```python
from build123d import *

# Parameters (mm, degrees)
BOX548_W               = 15
BOX548_H               = 13
BOX548_DEPTH           = 4.5
BOX548_ROLL_ANGLE      = 45
CYLINDER061_R          = 1.2
CYLINDER061_DEPTH      = 20
CYLINDER064_R          = 2
CYLINDER064_DEPTH      = 5
CYLINDER063_R          = 2
CYLINDER063_DEPTH      = 5
CYLINDER060_R          = 1.2
CYLINDER060_DEPTH      = 20
CYLINDER059_R          = 1.25
CYLINDER059_DEPTH      = 4.5
CYLINDER052_R          = 3.5
CYLINDER052_DEPTH      = 4.5
BOX043_W               = 7
BOX043_H               = 7.5
BOX043_DEPTH           = 5
BOX044_W               = 7
BOX044_H               = 7.5
BOX044_DEPTH           = 5
BOX041_W               = 8
BOX041_H               = 25
BOX041_DEPTH           = 4.5
CYLINDER053_R          = 5
CYLINDER053_DEPTH      = 4.5
FILLET011_R            = 3.99
BOX042_W               = 43
BOX042_H               = 7.5
BOX042_DEPTH           = 4.5
CHAMFER003_SIZE        = 6
FILLET012_R            = 3.5
CUT073_PLACEMENT_ANGLE = 180


with BuildPart() as cube739:
    # Box548 → Box548 (new body)
    with BuildSketch(Plane.XY):
        with Locations((7.5, 6.5)):
            Rectangle(BOX548_W, BOX548_H)
    extrude(amount=BOX548_DEPTH)


with BuildPart() as cube739_1:
    # Box548 roll: moved
    add(cube739.part.rotate(Axis((0, 0, 0), (1, 0, 0)), BOX548_ROLL_ANGLE))


with BuildPart() as cube739_2:
    # Box548 placement: moved
    add(cube739_1.part.moved(Location((90, 10, -34.25))))


with BuildPart() as cylinder061:
    # Cylinder061 → Cylinder061 (new body)
    with BuildSketch(Plane(origin=(-18.5, -4.75, -9.7), x_dir=(1, 0, 0), z_dir=(0, 0, 1))):
        Circle(CYLINDER061_R)
    extrude(amount=CYLINDER061_DEPTH)


with BuildPart() as fusion040:
    # Cylinder064 → Cylinder064 (new body)
    with BuildSketch(Plane(origin=(-18.5, -4.75, -9.2), x_dir=(1, 0, 0), z_dir=(0, 0, 1))):
        Circle(CYLINDER064_R)
    extrude(amount=CYLINDER064_DEPTH)

    # Fusion040: union Cylinder061
    add(cylinder061.part)


with BuildPart() as cylinder063:
    # Cylinder063 → Cylinder063 (new body)
    with BuildSketch(Plane(origin=(17.5, -4.75, -9.2), x_dir=(1, 0, 0), z_dir=(0, 0, 1))):
        Circle(CYLINDER063_R)
    extrude(amount=CYLINDER063_DEPTH)


with BuildPart() as fusion041:
    # Cylinder060 → Cylinder060 (new body)
    with BuildSketch(Plane(origin=(17.5, -4.75, -9.7), x_dir=(1, 0, 0), z_dir=(0, 0, 1))):
        Circle(CYLINDER060_R)
    extrude(amount=CYLINDER060_DEPTH)

    # Fusion039: union Cylinder063
    add(cylinder063.part)

    # Fusion041: union Fusion040
    add(fusion040.part)


with BuildPart() as cylinder059:
    # Cylinder059 → Cylinder059 (new body)
    with BuildSketch(Plane(origin=(0, -21, -9.2), x_dir=(1, 0, 0), z_dir=(0, 0, 1))):
        Circle(CYLINDER059_R)
    extrude(amount=CYLINDER059_DEPTH)


with BuildPart() as cylinder052:
    # Cylinder052 → Cylinder052 (new body)
    with BuildSketch(Plane.XY.offset(-9.2)):
        Circle(CYLINDER052_R)
    extrude(amount=CYLINDER052_DEPTH)


with BuildPart() as cube003:
    # Box043 → Box043 (new body)
    with BuildSketch(Plane(origin=(-22, -8.5, -4.7), x_dir=(1, 0, 0), z_dir=(0, 0, 1))):
        with Locations((3.5, 3.75)):
            Rectangle(BOX043_W, BOX043_H)
    extrude(amount=BOX043_DEPTH)


with BuildPart() as cube004:
    # Box044 → Box044 (new body)
    with BuildSketch(Plane(origin=(14, -8.5, -4.7), x_dir=(1, 0, 0), z_dir=(0, 0, 1))):
        with Locations((3.5, 3.75)):
            Rectangle(BOX044_W, BOX044_H)
    extrude(amount=BOX044_DEPTH)


with BuildPart() as cube001:
    # Box041 → Box041 (new body)
    with BuildSketch(Plane(origin=(-4, -25, -9.2), x_dir=(1, 0, 0), z_dir=(0, 0, 1))):
        with Locations((4, 12.5)):
            Rectangle(BOX041_W, BOX041_H)
    extrude(amount=BOX041_DEPTH)


with BuildPart() as fillet011:
    # Cylinder053 → Cylinder053 (new body)
    with BuildSketch(Plane.XY.offset(-9.2)):
        Circle(CYLINDER053_R)
    extrude(amount=CYLINDER053_DEPTH)

    # Fusion034: union Cube001
    add(cube001.part)

    # Fillet011
    fillet011_edges = [fillet011.edges().sort_by_distance(p)[0] for p in [
        (4, -25, -6.95),
        (-4, -25, -6.95),
    ]]
    fillet(fillet011_edges, radius=FILLET011_R)


with BuildPart() as obj1:
    # Box042 → Box042 (new body)
    with BuildSketch(Plane(origin=(-22, -8.5, -9.2), x_dir=(1, 0, 0), z_dir=(0, 0, 1))):
        with Locations((21.5, 3.75)):
            Rectangle(BOX042_W, BOX042_H)
    extrude(amount=BOX042_DEPTH)

    # Fusion036: union Cube003, Cube004, Fillet011
    add(cube003.part)
    add(cube004.part)
    add(fillet011.part)

    # Cut066: cut Cylinder052
    add(cylinder052.part, mode=Mode.SUBTRACT)

    # Chamfer003
    chamfer003_edges = [obj1.edges().sort_by_distance(p)[0] for p in [
        (21, -4.75, -9.2),
        (-22, -4.75, -9.2),
    ]]
    chamfer(chamfer003_edges, length=CHAMFER003_SIZE)

    # Fillet012
    fillet012_edges = [obj1.edges().sort_by_distance(p)[0] for p in [
        (-22, -8.5, -1.45),
        (-22, -1, -1.45),
        (21, -1, -1.45),
        (21, -8.5, -1.45),
    ]]
    fillet(fillet012_edges, radius=FILLET012_R)

    # Cut067: cut Cylinder059
    add(cylinder059.part, mode=Mode.SUBTRACT)

    # Cut073: cut Fusion041
    add(fusion041.part, mode=Mode.SUBTRACT)


with BuildPart() as obj1_1:
    # Cut073 placement: moved
    add(obj1.part.moved(Location((98, 16.5, -39))).rotate(Axis((98, 16.5, -39), (1, 0, 0)), CUT073_PLACEMENT_ANGLE))

    # Cut670: cut Cube739
    add(cube739_2.part, mode=Mode.SUBTRACT)


solid = obj1_1.part
```
Check sheet for the modelled part. Datum: model origin and axes. Units: mm. A direction names the side the tool comes from. Give positions to 0.01 mm unless a question says otherwise; leave off trailing zeros. Write each loop counter-clockwise with the first axis right and the second up, starting at its lowest first coordinate (ties: lowest second). Pieces come first, ordered by that corner, then holes. Notation, with made-up numbers: (46, 29) - (64, 29) arc R20 cw to (64, 37) - close; hole circle Ø5 at (80.25, 11). An arc over 180 degrees is marked (long way). Answer as a JSON object with one key per item and string values. Group by question number.
1) Sectioned sample at D-D (x = 91.5). Record the cut outline in (y, z).
2) Depth check by flat-ended pin: P1, Ø14.5, axis at x = 103.5, y = 31, coming from the -Z side; P2, Ø3, axis at x = 87, z = -32.5, coming from the -Y side; P3, Ø5, axis at x = 91, z = -31, coming from the +Y side; P4, Ø6.5, axis at x = 98, y = 16.5, coming from the -Z side. Enter the tip coordinate at first touch or a pass-through.
3) Sectioned sample at A-A (y = 16.5). Record the cut outline in (x, z).
4) Sectioned sample at B-B (z = -35.25). Record the cut outline in (x, y).
5) Thickness scan on probe 1 along Y at (x, z) = (79.5, -36.1); probe 2 along X at (y, z) = (37.5, -33.25); probe 3 along Z at (x, y) = (97, 35.5). Record the ranges inside material, lowest first. Write a range as from..to.
6) Release check for a two-part mould opening along X. For faces 1 (the face through (97.94, 12.67, -31.58)), 2 (the face through (100.8, 40.36, -32.08)), 3 (the face through (79, 23, -34.8)), 4 (the face through (95.14, 40.3, -32.08)) record: pulls with the +X half, pulls with the -X half, needs draft (parallel to the pull), parting line crosses it, or undercut.
7) Sectioned sample at C-C (x = 115). Record the cut outline in (y, z).
8) Access from +Z, -Z, +X, -X, +Y, -Y to the whole of each face (thin tool, end or side, straight path). Record for faces 5 (the face through (112, 21, -37)), 6 (the face through (94, 31, -32)), 7 (the face through (102, 31, -32)).
Geometry results:
{
 "1": {"outline": "(17.5, -34.3) - (25, -34.3) - (25, -29.8) - (17.5, -29.8) - close"},
 "2": {"P1": "stops at z = -34.3", "P2": "stops at y = 17.5", "P3": "stops at y = 25", "P4": "passes through"},
 "3": {"outline": "(93, -34.3) - (94.5, -34.3) - (94.5, -29.8) - (93, -29.8) - close; (101.5, -34.3) - (103, -34.3) - (103, -29.8) - (101.5, -29.8) - close"},
 "4": {"outline": "(76.55, 19.12) arc R3.5 ccw to (79.5, 17.5) - (83, 17.5) - (83, 25) - (79.5, 25) arc R3.5 ccw to (76.55, 23.38) - close; (112, 17.5) - (115.5, 17.5) arc R3.5 ccw to (118.45, 19.12) - (118.45, 23.38) arc R3.5 ccw to (115.5, 25) - (112, 25) - close; hole circle Ø2.4 at (79.5, 21.25); hole circle Ø2.4 at (115.5, 21.25)"},
 "5": {"probe 1": "y = 17.5..20.05, 22.45..25", "probe 2": "x = 94..96.75, 99.25..102", "probe 3": "z = -34.3..-29.8"},
 "6": {"face 1": "needs draft", "face 2": "pulls with the +X half", "face 3": "undercut", "face 4": "pulls with the -X half"},
 "7": {"outline": "(17.5, -39.3) - (20.16, -39.3) - (20.16, -34.8) - (19.31, -34.8) - (19.31, -31.8) - (17.5, -31.8) - close; (22.34, -39.3) - (25, -39.3) - (25, -31.8) - (23.19, -31.8) - (23.19, -34.8) - (22.34, -34.8) - close"},
 "8": {"face 5": "-Z, +Y, -Y", "face 6": "+Z, -Z, -X, +Y", "face 7": "+Z, -Z, +X, +Y"}
}
